Geometry: final body of the model. Coordinates: model frame, mm. A direction names the side the tool comes from. Coordinates: 2 decimals unless noted, no trailing zeros. Loops run counter-clockwise (first coordinate to the right, second up) from the corner with the lowest first, then second, coordinate; pieces in that order, holes last. Notation, with made-up numbers: (65.25, -8) - (86.25, -8) arc R23 ccw to (86.25, 11) - close; hole circle Ø5 at (44, 12). An arc over 180 degrees is marked (long way). Answer in a Markdown table with one row per item.
from build123d import *

# Parameters (mm, degrees)
CROQUIS1_W                                 = 56.1
CROQUIS1_H                                 = 56.1
SALIENTE_EXTRUIR1_DEPTH                    = 76.05
CORTAR_EXTRUIR1_DEPTH                      = 82.199307
SIMETR_A3_AT_THE_SECOND_PLANE_COPY_1_DEPTH = 82.199307
CHAFL_N1_SIZE                              = 2.5
CROQUIS3_R                                 = 2.25
CORTAR_EXTRUIR2_DEPTH                      = 82.199307
SIMETR_A4_AT_THE_SECOND_PLANE_COPY_1_SKE_R = 2.25
SIMETR_A4_AT_THE_SECOND_PLANE_COPY_1_DEPTH = 82.199307
CROQUIS4_R                                 = 19.25
SALIENTE_EXTRUIR2_DEPTH                    = 2.5
CROQUIS6_R                                 = 3.5
SALIENTE_EXTRUIR4_DEPTH                    = 11.7
SALIENTE_EXTRUIR5_DEPTH                    = 28.15
SALIENTE_EXTRUIR3_DEPTH                    = 39.95


with BuildPart() as part:
    # Croquis1 → Saliente-Extruir1 (new body)
    with BuildSketch(Plane(origin=(0, 0, 0), x_dir=(1, 0, 0), z_dir=(0, 1, 0))):
        Rectangle(CROQUIS1_W, CROQUIS1_H)
    extrude(amount=SALIENTE_EXTRUIR1_DEPTH)

    # Croquis2 → Cortar-Extruir1 (cut, through all)
    with BuildSketch(Plane(origin=(0, 70.85, 0), x_dir=(1, 0, 0), z_dir=(0, 1, 0))):
        with BuildLine():
            Line((-28.05, 19.7), (-23.875, 19.7))
            ThreePointArc((-23.875, 19.7), (-20.922829, 20.922829), (-19.7, 23.875))
            Line((-19.7, 23.875), (-19.7, 28.05))
            Line((-19.7, 28.05), (-28.05, 28.05))
            Line((-28.05, 28.05), (-28.05, 19.7))
        make_face()
    cortar_extruir1 = extrude(amount=-CORTAR_EXTRUIR1_DEPTH, mode=Mode.SUBTRACT)

    # Simetría3: Cortar-Extruir1 across plane
    add(cortar_extruir1.mirror(Plane(origin=(0, 0, 0), x_dir=(0, 0, 1), z_dir=(1, 0, 0))), mode=Mode.SUBTRACT)

    # Simetría3 at the second plane: Cortar-Extruir1 across plane
    add(cortar_extruir1.mirror(Plane.XY), mode=Mode.SUBTRACT)

    # Simetría3 at the second plane copy 1 ske → Simetría3 at the second plane copy 1 (cut, through all)
    with BuildSketch(Plane(origin=(0, 70.85, 0), x_dir=(-1, 0, 0), z_dir=(0, 1, 0))):
        with BuildLine():
            Line((-28.05, 19.7), (-23.875, 19.7))
            ThreePointArc((-23.875, 19.7), (-20.922829, 20.922829), (-19.7, 23.875))
            Line((-19.7, 23.875), (-19.7, 28.05))
            Line((-19.7, 28.05), (-28.05, 28.05))
            Line((-28.05, 28.05), (-28.05, 19.7))
        make_face()
    extrude(amount=-SIMETR_A3_AT_THE_SECOND_PLANE_COPY_1_DEPTH, mode=Mode.SUBTRACT)

    # Chaflán1
    chafl_n1_edges = [part.edges().sort_by_distance(p)[0] for p in [
        (-28.05, 35.425, -19.7),
        (-19.7, 35.425, -28.05),
        (-28.05, 35.425, 19.7),
        (-19.7, 35.425, 28.05),
        (28.05, 35.425, -19.7),
        (19.7, 35.425, -28.05),
        (28.05, 35.425, 19.7),
        (19.7, 35.425, 28.05),
    ]]
    chamfer(chafl_n1_edges, length=CHAFL_N1_SIZE)

    # Croquis3 → Cortar-Extruir2 (cut, through all)
    with BuildSketch(Plane.XZ.offset(-70.85)):
        with Locations(Location((23.875, -23.875, 0), (0, 0, 270))):
            Circle(CROQUIS3_R)
    cortar_extruir2 = extrude(amount=-CORTAR_EXTRUIR2_DEPTH, mode=Mode.SUBTRACT)

    # Simetría4: Cortar-Extruir2 across plane
    add(cortar_extruir2.mirror(Plane(origin=(0, 0, 0), x_dir=(0, 0, 1), z_dir=(1, 0, 0))), mode=Mode.SUBTRACT)

    # Simetría4 at the second plane: Cortar-Extruir2 across plane
    add(cortar_extruir2.mirror(Plane.XY), mode=Mode.SUBTRACT)

    # Simetría4 at the second plane copy 1 ske → Simetría4 at the second plane copy 1 (cut, through all)
    with BuildSketch(Plane(origin=(0, 70.85, 0), x_dir=(-1, 0, 0), z_dir=(0, -1, 0))):
        with Locations(Location((23.875, -23.875, 0), (0, 0, 270))):
            Circle(SIMETR_A4_AT_THE_SECOND_PLANE_COPY_1_SKE_R)
    extrude(amount=-SIMETR_A4_AT_THE_SECOND_PLANE_COPY_1_DEPTH, mode=Mode.SUBTRACT)

    # Croquis4 → Saliente-Extruir2 (add)
    with BuildSketch(Plane(origin=(0, 76.05, 0), x_dir=(1, 0, 0), z_dir=(0, 1, 0))):
        with Locations(Location((0, 0, 0), (0, 0, 270))):
            Circle(CROQUIS4_R)
    extrude(amount=SALIENTE_EXTRUIR2_DEPTH)

    # Croquis6 → Saliente-Extruir4 (add)
    with BuildSketch(Plane(origin=(0, 78.55, 0), x_dir=(1, 0, 0), z_dir=(0, 1, 0))):
        with Locations(Location((0, 0, 0), (0, 0, 270))):
            Circle(CROQUIS6_R)
    extrude(amount=SALIENTE_EXTRUIR4_DEPTH)

    # Croquis7 → Saliente-Extruir5 (add)
    with BuildSketch(Plane(origin=(0, 90.25, 0), x_dir=(1, 0, 0), z_dir=(0, 1, 0))):
        with BuildLine():
            Line((-2.397394, 2.55), (2.397394, 2.55))
            ThreePointArc((2.397394, 2.55), (0, -3.5), (-2.397394, 2.55))
        make_face()
    extrude(amount=SALIENTE_EXTRUIR5_DEPTH)

    # Croquis5 → Saliente-Extruir3 (add)
    with BuildSketch(Plane(origin=(0, 78.55, 0), x_dir=(1, 0, 0), z_dir=(0, 1, 0))):
        with BuildLine():
            Line((-2.397394, 2.55), (2.397394, 2.55))
            ThreePointArc((2.397394, 2.55), (0, -3.5), (-2.397394, 2.55))
        make_face()
    extrude(amount=SALIENTE_EXTRUIR3_DEPTH)


solid = part.part
(1) Pull-direction query (X, two-part tool) for faces 1 (the face through (23.9, 70.85, -26.3)), 2 (the face through (28.05, 37, 0)), 3 (the face through (21.879, 73.414, -24.913)); classes: pulls with the +X half, pulls with the -X half, needs draft (parallel to the pull), parting line crosses it, or undercut.
Verdict:
| item | result |
|---|---|
| face 1 | needs draft |
| face 2 | pulls with the +X half |
| face 3 | undercut |
(2) Cut plane C-C on y = 32. Output: boundary loops of the cut face in (x, z) (3 decimals), then the cut area to 3 significant figures.
Verdict:
| item | result |
|---|---|
| outline | (-28.05, -17.2) - (-25.55, -19.7) - (-23.875, -19.7) arc R4.175 cw to (-19.7, -23.875) - (-19.7, -25.55) - (-17.2, -28.05) - (17.2, -28.05) - (19.7, -25.55) - (19.7, -23.875) arc R4.175 cw to (23.875, -19.7) - (25.55, -19.7) - (28.05, -17.2) - (28.05, 17.2) - (25.55, 19.7) - (23.875, 19.7) arc R4.175 cw to (19.7, 23.875) - (19.7, 25.55) - (17.2, 28.05) - (-17.2, 28.05) - (-19.7, 25.55) - (-19.7, 23.875) arc R4.175 cw to (-23.875, 19.7) - (-25.55, 19.7) - (-28.05, 17.2) - close |
| area | 2,860 mm² |
(3) Access query for faces 4 (the face through (-7, 76.05, -19)), 5 (the face through (26.82, 35.92, -18.43)), 6 (the face through (20.955, 35.921, 20.891)), 7 (the face through (-23.9, 70.85, 26.3)). Directions: +Z, -Z, +X, -X, +Y, -Y. A direction counts if a zero-diameter tool reaches every point of the face in a straight line with its end or side. Return the directions, or none.
Verdict:
| item | result |
|---|---|
| face 4 | +Y |
| face 5 | -Z, +X, -Y |
| face 6 | +Z, +X, -Y |
| face 7 | +Z, -X, -Y |
(4) First-contact query: pin 1 Ø0.8 at (x, y) = (25, 23.5) entering from -Z; pin 2 Ø4 at (x, y) = (-4.5, 82) entering from +Z; pin 3 Ø3.5 at (x, z) = (23, -23) entering from -Y. Flat tips, straight axial feed; report the tip coordinate or a pass-through.
Verdict:
| item | result |
|---|---|
| pin 1 | stops at z = -19.7 |
| pin 2 | stops at z = 2.45 |
| pin 3 | stops at y = 70.85 |
(5) Cut plane A-A on z = 0. Output: boundary loops of the cut face in (x, y), then the cut area to 3 significant figures.
Verdict:
| item | result |
|---|---|
| outline | (-28.05, 0) - (28.05, 0) - (28.05, 76.05) - (19.25, 76.05) - (19.25, 78.55) - (3.5, 78.55) - (3.5, 118.5) - (-3.5, 118.5) - (-3.5, 78.55) - (-19.25, 78.55) - (-19.25, 76.05) - (-28.05, 76.05) - close |
| area | 4,640 mm² |
(6) Ray query, probe 1 along Y at (x, z) = (-23.5, 20); probe 2 along Y at (x, z) = (19, 6.5); probe 3 along X at (y, z) = (64.5, -23.5). Return the intervals inside material, ascending.
Verdict:
| item | result |
|---|---|
| probe 1 | y = 70.85 to 76.05 |
| probe 2 | y = 0 to 76.05 |
| probe 3 | x = -19.72 to 19.72 |
(7) Cut plane B-B on x = 0. Output: boundary loops of the cut face in (y, z).
Verdict:
| item | result |
|---|---|
| outline | (0, -28.05) - (76.05, -28.05) - (76.05, -19.25) - (78.55, -19.25) - (78.55, -3.5) - (90.25, -3.5) - (90.25, -2.55) - (118.5, -2.55) - (118.5, 3.5) - (78.55, 3.5) - (78.55, 19.25) - (76.05, 19.25) - (76.05, 28.05) - (0, 28.05) - close |
(8) Cut plane D-D on x = 10. Output: boundary loops of the cut face in (y, z), then the cut area to 3 significant figures.
Verdict:
| item | result |
|---|---|
| outline | (0, -28.05) - (76.05, -28.05) - (76.05, -16.45) - (78.55, -16.45) - (78.55, 16.45) - (76.05, 16.45) - (76.05, 28.05) - (0, 28.05) - close |
| area | 4,350 mm² |
